Can you work these out from the drawing? Everything is in mm from the part's minimum corner. A direction names the side the tool comes from. Round coordinates to 2 decimals unless told otherwise and drop trailing zeros. Loops run counter-clockwise (first coordinate to the right, second up) from the corner with the lowest first, then second, coordinate; pieces in that order, holes last. Notation, with made-up numbers: (10.25, 38) -> (60.25, 38) arc R26 ccw to (60.25, 55) -> close; hole circle Ø1 at (-13.75, 75.5). An arc over 180 degrees is marked (long way). One line per item, written item: value.
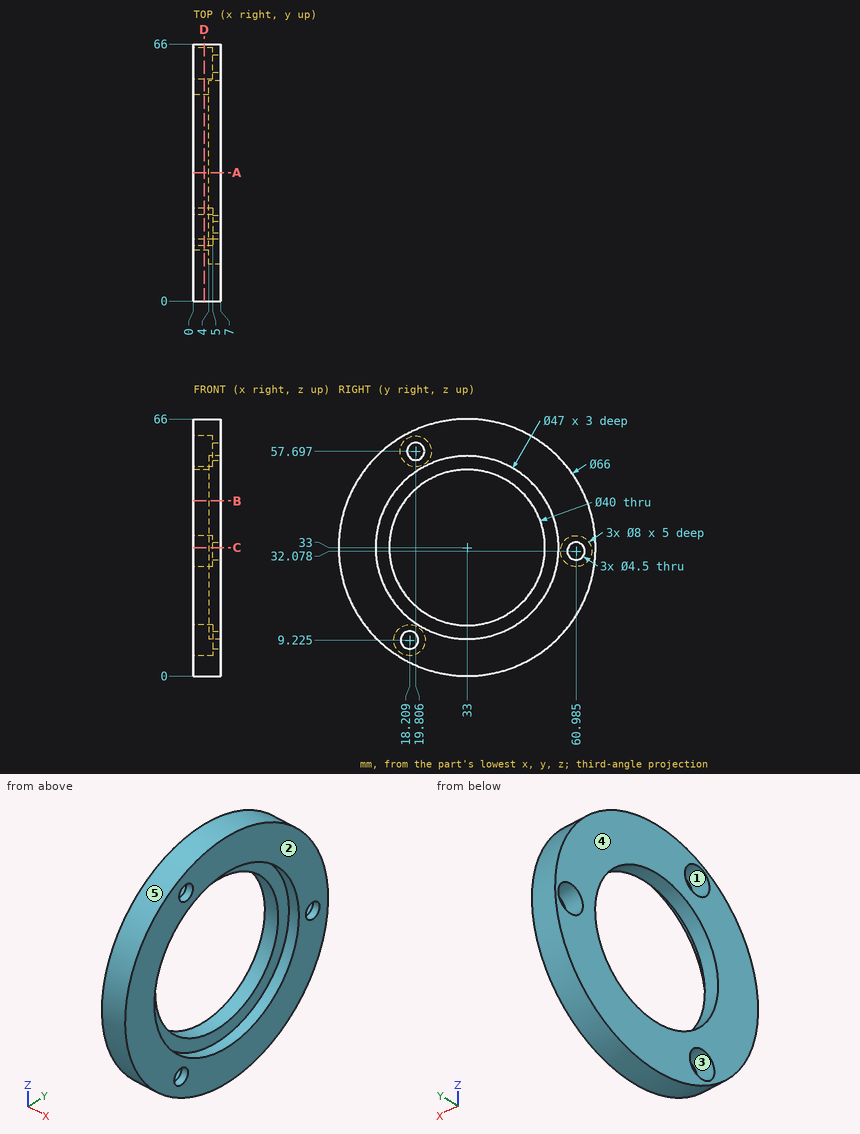
(1) Imagine slicing it at A-A on y = 33. Write out the boundary of the cut face in (x, z).
Results below:
outline: (0, 0) -> (7, 0) -> (7, 9.5) -> (4, 9.5) -> (4, 13) -> (0, 13) -> close; (0, 53) -> (4, 53) -> (4, 56.5) -> (7, 56.5) -> (7, 66) -> (0, 66) -> close
(2) We'd pull the mould along Z, two halves only. Please class the marked faces 3, 4 and 5: +Z half, -Z half, draft (parallel to the pull), parting line (faces both ways), or undercut.
Results below:
face 3: undercut
face 4: draft
face 5: parting line
(3) For pin 1 Ø1.5 at (x, z) = (4.5, 48.5) entering from -Y; pin 2 Ø5 at (y, z) = (7, 56.5) entering from +X; pin 3 Ø2.5 at (y, z) = (21, 57) entering from -X; pin 4 Ø4 at (x, y) = (5.5, 20) entering from -Z, each with a flat end and sliding along its axis, tell me the tip position at first contact or that it passes through.
Results below:
pin 1: stops at y = 3.48
pin 2: stops at x = 7
pin 3: stops at x = 5
pin 4: stops at z = 1.89
(4) On a 3-axis mill with a long thin cutter (end or side, diameter ignored), from which of +Z, -Z, +X, -X, +Y, -Y can I reach the whole of each face in a straight line? I mean the marked faces 1 and 2. Say none if no direction works.
Results below:
face 1: -X
face 2: +Z, -Z, +X, +Y, -Y
(5) Imagine slicing it at C-C on z = 33. Write out the boundary of the cut face in (x, y), then the cut area to 3 significant figures.
Results below:
outline: (0, 0) -> (7, 0) -> (7, 9.5) -> (4, 9.5) -> (4, 13) -> (0, 13) -> close; (0, 53) -> (4, 53) -> (4, 56.5) -> (7, 56.5) -> (7, 58.93) -> (5, 58.93) -> (5, 57.09) -> (0, 57.09) -> close; (0, 64.88) -> (5, 64.88) -> (5, 63.04) -> (7, 63.04) -> (7, 66) -> (0, 66) -> close
area: 114 mm²
(6) Imagine slicing it at D-D on x = 2.75. Write out the boundary of the cut face in (y, z) (1 decimal).
Results below:
outline: circle Ø66 at (33, 33); hole circle Ø40 at (33, 33); hole circle Ø8 at (18.2, 9.2); hole circle Ø8 at (19.8, 57.7); hole circle Ø8 at (61, 32.1)
(7) Imagine slicing it at B-B on z = 45. Write out the boundary of the cut face in (x, y) (1 decimal), then the cut area to 3 significant figures.
Results below:
outline: (0, 2.3) -> (7, 2.3) -> (7, 12.8) -> (4, 12.8) -> (4, 17) -> (0, 17) -> close; (0, 49) -> (4, 49) -> (4, 53.2) -> (7, 53.2) -> (7, 63.7) -> (0, 63.7) -> close
area: 181 mm²
(8) Please list where these lines run through material, in increasing order: L1, parallel to X at y = 24.5, z = 11.5; L2, parallel to Y at x = 4, z = 58.5 (1 decimal); L3, parallel to Y at x = 6.25, z = 54.5 (1 decimal).
Results below:
L1: x = 0 to 4
L2: y = 12.1 to 15.9, 23.7 to 53.9
L3: y = 8 to 23.5, 42.5 to 58
